The model under review builds one solid part; all positions refer to its coordinate system, in mm. Give positions to 0.01 mm unless a question says otherwise; leave off trailing zeros. Answer as a JSON object with one key per item and string values.
Autodesk Inventor part; units mm, degrees
ref_plane "YZ Plane" through (0, 0, 0) normal (1, 0, 0) x (0, 1, 0)
ref_plane "XZ Plane" through (0, 0, 0) normal (0, 1, 0) x (-1, 0, 0)
ref_plane "XY Plane" through (0, 0, 0) normal (0, 0, 1) x (1, 0, 0)
sketch "Sketch1" plane through (0, 0, 0) normal (1, 0, 0) x (0, 1, 0)
  line L0 (9.5486, -7.0751) -> (4.5486, -7.0751)
  line L1 (7.0486, -9.5751) -> (7.0486, -4.5751)
  circle A0 centre (7.0486, -7.0751) radius 2
  circle A1 centre (7.0486, 6.9249) radius 2
  line L2 (7.0486, 9.4249) -> (7.0486, 4.4249)
  line L3 (9.5486, 6.9249) -> (4.5486, 6.9249)
  line L4 (4.1986, 4.8676) -> (4.1986, 8.1249)
  arc A2 (4.1986, 8.1249) -> (3.8986, 8.4249) centre (3.8986, 8.1249) ccw
  line L5 (3.8986, 8.4249) -> (2.9986, 8.4249)
  arc A3 (2.6986, 8.7249) -> (2.9986, 8.4249) centre (2.9986, 8.7249) ccw
  line L6 (2.6986, 8.7249) -> (2.6986, 9.6249)
  arc A4 (2.9986, 9.9249) -> (2.6986, 9.6249) centre (2.9986, 9.6249) ccw
  line L7 (2.9986, 9.9249) -> (9.7486, 9.9249)
  arc A5 (10.0486, 9.6249) -> (9.7486, 9.9249) centre (9.7486, 9.6249) ccw
  line L8 (10.0486, 9.6249) -> (10.0486, 2.8749)
  arc A6 (9.7486, 2.5749) -> (10.0486, 2.8749) centre (9.7486, 2.8749) ccw
  line L9 (9.7486, 2.5749) -> (8.8486, 2.5749)
  arc A7 (8.5486, 2.8749) -> (8.8486, 2.5749) centre (8.8486, 2.8749) ccw
  line L10 (8.5486, 2.8749) -> (8.5486, 3.7749)
  arc A8 (8.5486, 3.7749) -> (8.2486, 4.0749) centre (8.2486, 3.7749) ccw
  line L11 (8.2486, 4.0749) -> (4.9914, 4.0749)
  arc A9 (4.9914, 4.0749) -> (4.7564, 3.9614) centre (4.9914, 3.7749) ccw
  arc A10 (4.7564, 3.9614) -> (3.3559, 0.2322) centre (9.8395, -0.0751) ccw
  line L12 (3.3559, 0.2322) -> (3.0486, -0.0751)
  line L13 (3.0486, -0.0751) -> (3.3559, -0.3824)
  arc A11 (3.3559, -0.3824) -> (4.7564, -4.1117) centre (9.8395, -0.0751) ccw
  arc A12 (4.7564, -4.1117) -> (4.9914, -4.2251) centre (4.9914, -3.9251) ccw
  line L14 (4.9914, -4.2251) -> (8.2486, -4.2251)
  arc A13 (8.2486, -4.2251) -> (8.5486, -3.9251) centre (8.2486, -3.9251) ccw
  line L15 (8.5486, -3.9251) -> (8.5486, -3.0251)
  arc A14 (8.8486, -2.7251) -> (8.5486, -3.0251) centre (8.8486, -3.0251) ccw
  line L16 (8.8486, -2.7251) -> (9.7486, -2.7251)
  arc A15 (10.0486, -3.0251) -> (9.7486, -2.7251) centre (9.7486, -3.0251) ccw
  line L17 (10.0486, -3.0251) -> (10.0486, -9.7751)
  arc A16 (9.7486, -10.0751) -> (10.0486, -9.7751) centre (9.7486, -9.7751) ccw
  line L18 (9.7486, -10.0751) -> (2.9986, -10.0751)
  arc A17 (2.6986, -9.7751) -> (2.9986, -10.0751) centre (2.9986, -9.7751) ccw
  line L19 (2.6986, -9.7751) -> (2.6986, -8.8751)
  arc A18 (2.9986, -8.5751) -> (2.6986, -8.8751) centre (2.9986, -8.8751) ccw
  line L20 (2.9986, -8.5751) -> (3.8986, -8.5751)
  arc A19 (3.8986, -8.5751) -> (4.1986, -8.2751) centre (3.8986, -8.2751) ccw
  line L21 (4.1986, -8.2751) -> (4.1986, -5.0179)
  arc A20 (4.1986, -5.0179) -> (4.0852, -4.7829) centre (3.8986, -5.0179) ccw
  arc A21 (4.0852, -4.7829) -> (0.3559, -3.3824) centre (0.0486, -9.8659) ccw
  line L22 (0.3559, -3.3824) -> (0.0486, -3.0751)
  line L23 (0.0486, -3.0751) -> (-0.2587, -3.3824)
  arc A22 (-0.2587, -3.3824) -> (-3.9879, -4.7829) centre (0.0486, -9.8659) ccw
  arc A23 (-3.9879, -4.7829) -> (-4.1014, -5.0179) centre (-3.8014, -5.0179) ccw
  line L24 (-4.1014, -5.0179) -> (-4.1014, -8.2751)
  arc A24 (-4.1014, -8.2751) -> (-3.8014, -8.5751) centre (-3.8014, -8.2751) ccw
  line L25 (-3.8014, -8.5751) -> (-2.9014, -8.5751)
  arc A25 (-2.6014, -8.8751) -> (-2.9014, -8.5751) centre (-2.9014, -8.8751) ccw
  line L26 (-2.6014, -8.8751) -> (-2.6014, -9.7751)
  arc A26 (-2.9014, -10.0751) -> (-2.6014, -9.7751) centre (-2.9014, -9.7751) ccw
  line L27 (-2.9014, -10.0751) -> (-9.6514, -10.0751)
  arc A27 (-9.9514, -9.7751) -> (-9.6514, -10.0751) centre (-9.6514, -9.7751) ccw
  line L28 (-9.9514, -9.7751) -> (-9.9514, -3.0251)
  arc A28 (-9.6514, -2.7251) -> (-9.9514, -3.0251) centre (-9.6514, -3.0251) ccw
  line L29 (-9.6514, -2.7251) -> (-8.7514, -2.7251)
  arc A29 (-8.4514, -3.0251) -> (-8.7514, -2.7251) centre (-8.7514, -3.0251) ccw
  line L30 (-8.4514, -3.0251) -> (-8.4514, -3.9251)
  arc A30 (-8.4514, -3.9251) -> (-8.1514, -4.2251) centre (-8.1514, -3.9251) ccw
  line L31 (-8.1514, -4.2251) -> (-4.8941, -4.2251)
  arc A31 (-4.8941, -4.2251) -> (-4.6592, -4.1117) centre (-4.8941, -3.9251) ccw
  arc A32 (-4.6592, -4.1117) -> (-3.2587, -0.3824) centre (-9.7422, -0.0751) ccw
  line L32 (-3.2587, -0.3824) -> (-2.9514, -0.0751)
  line L33 (-2.9514, -0.0751) -> (-3.2587, 0.2322)
  arc A33 (-3.2587, 0.2322) -> (-4.6592, 3.9614) centre (-9.7422, -0.0751) ccw
  arc A34 (-4.6592, 3.9614) -> (-4.8941, 4.0749) centre (-4.8941, 3.7749) ccw
  line L34 (-4.8941, 4.0749) -> (-8.1514, 4.0749)
  arc A35 (-8.1514, 4.0749) -> (-8.4514, 3.7749) centre (-8.1514, 3.7749) ccw
  line L35 (-8.4514, 3.7749) -> (-8.4514, 2.8749)
  arc A36 (-8.7514, 2.5749) -> (-8.4514, 2.8749) centre (-8.7514, 2.8749) ccw
  line L36 (-8.7514, 2.5749) -> (-9.6514, 2.5749)
  arc A37 (-9.9514, 2.8749) -> (-9.6514, 2.5749) centre (-9.6514, 2.8749) ccw
  line L37 (-9.9514, 2.8749) -> (-9.9514, 9.6249)
  arc A38 (-9.6514, 9.9249) -> (-9.9514, 9.6249) centre (-9.6514, 9.6249) ccw
  line L38 (-9.6514, 9.9249) -> (-2.9014, 9.9249)
  arc A39 (-2.6014, 9.6249) -> (-2.9014, 9.9249) centre (-2.9014, 9.6249) ccw
  line L39 (-2.6014, 9.6249) -> (-2.6014, 8.7249)
  arc A40 (-2.9014, 8.4249) -> (-2.6014, 8.7249) centre (-2.9014, 8.7249) ccw
  line L40 (-2.9014, 8.4249) -> (-3.8014, 8.4249)
  arc A41 (-3.8014, 8.4249) -> (-4.1014, 8.1249) centre (-3.8014, 8.1249) ccw
  line L41 (-4.1014, 8.1249) -> (-4.1014, 4.8676)
  arc A42 (-4.1014, 4.8676) -> (-3.9879, 4.6327) centre (-3.8014, 4.8676) ccw
  arc A43 (-3.9879, 4.6327) -> (-0.2587, 3.2322) centre (0.0486, 9.7157) ccw
  line L42 (-0.2587, 3.2322) -> (0.0486, 2.9249)
  line L43 (0.0486, 2.9249) -> (0.3559, 3.2322)
  arc A44 (0.3559, 3.2322) -> (4.0852, 4.6327) centre (0.0486, 9.7157) ccw
  arc A45 (4.0852, 4.6327) -> (4.1986, 4.8676) centre (3.8986, 4.8676) ccw
  line L44 (-11.1503, -0.0751) -> (11.2475, -0.0751)
  circle A46 centre (0.0486, -0.0751) radius 2.15
  circle A47 centre (-6.9514, -7.0751) radius 2
  line L45 (-6.9514, -9.5751) -> (-6.9514, -4.5751)
  line L46 (-9.4514, -7.0751) -> (-4.4514, -7.0751)
  circle A48 centre (-6.9514, 6.9249) radius 2
  line L47 (-6.9514, 9.4249) -> (-6.9514, 4.4249)
  line L48 (-9.4514, 6.9249) -> (-4.4514, 6.9249)
extrude "Extrusion1" add sketch "Sketch1" along normal blind 150
equation "\"BendRadius\" = Thickness"
equation "\"BendReliefWidth\" = Thickness"
equation "\"BendReliefDepth\" = 0.5 * Thickness"
equation "\"CornerReliefSize\" = 4 * Thickness"
equation "\"MinimumRemnant\" = 2 * Thickness"
equation "\"TransitionRadius\" = BendRadius"
equation "\"JacobiRadiusSize\" = BendRadius"
equation "\"GapSize\" = Thickness"
properties part number "150mm 2020"
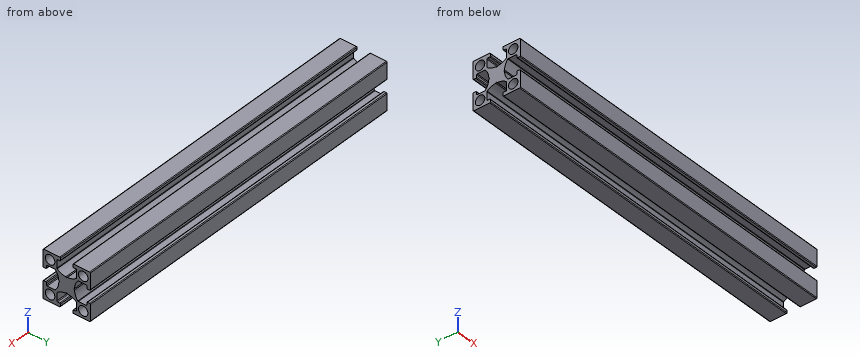
Q1. Consider section A-A, the plane x = 125. State how many separate pieces and enclosed holes the cut face has, plus the area to 3 significant figures.
Results:
{"separate pieces": "1", "enclosed holes": "4", "area": "160 mm^2"}
Q2. To check wall thickness, follow probe 1 along Y at (x, z) = (86, -3); probe 2 along Z at (x, y) = (110, 5.5); probe 3 along Y at (x, z) = (117, -6). State the ranges of each line that lie inside material, in increasing order. Write a range as [from, to].
Results:
{"probe 1": "y = [-9.95, -8.45], [-3.95, 4.04], [8.55, 10.05]", "probe 2": "z = [-10.08, -8.34], [-5.81, -4.23], [4.07, 5.66], [8.19, 9.92]", "probe 3": "y = [-9.95, -8.64], [-5.26, -4.1], [4.2, 5.36], [8.74, 10.05]"}
Q3. Clearance check with a flat-ended pin moving along its axis: pin 1 Ø10 at (y, z) = (2.5, -7.5) entering from +X. State where the tip first meets the part, or that it passes through.
Results:
{"pin 1": "stops at x = 150"}
